Geometry: final body of the model. Coordinates: model frame, mm. Face numbers are marked on the shaded views. Round coordinates to 2 decimals unless told otherwise and drop trailing zeros. Write each loop counter-clockwise with the first axis right and the second up, starting at its lowest first coordinate (ties: lowest second). Pieces come first, ordered by that corner, then holes. Notation, with made-up numbers: (-6.5, 44.25) - (7.5, 44.25) arc R18 cw to (7.5, 68.25) - close; hole circle Ø4 at (61, -4). An arc over 180 degrees is marked (long way). Use a Markdown table: item, result. Add a question column.
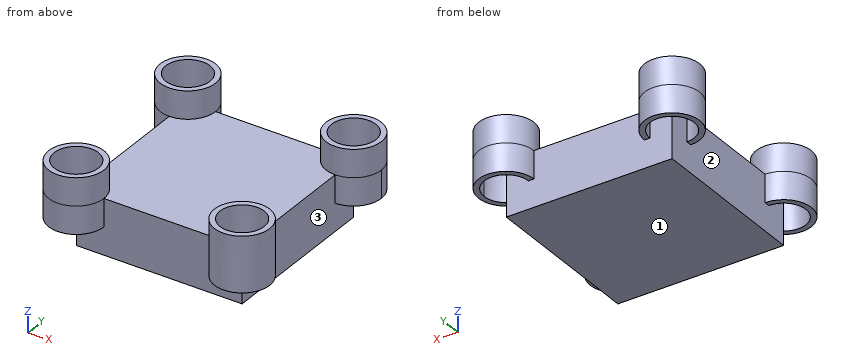
```python
from build123d import *

# Parameters (mm, degrees)
F0_W     = 76.2
F0_H     = 76.2
F1_DEPTH = 25.4
F2_R     = 12.7
F2_R_2   = 10.16
F3_DEPTH = 12.7


with BuildPart() as f1:
    # F0 (on Top) → F1 (new body)
    with BuildSketch(Plane.XY):
        Rectangle(F0_W, F0_H)
    extrude(amount=F1_DEPTH)

    # F2 (on face) → F3 (join, symmetric)
    with BuildSketch(Plane.XY.offset(25.4)):
        with Locations((-38.1, 38.1)):
            Circle(F2_R)
        with Locations((-38.1, 38.1)):
            Circle(F2_R_2, mode=Mode.SUBTRACT)
        with Locations((38.1, 38.1)):
            Circle(F2_R)
        with Locations((38.1, 38.1)):
            Circle(F2_R_2, mode=Mode.SUBTRACT)
        with Locations((-38.1, -38.1)):
            Circle(F2_R)
        with Locations((-38.1, -38.1)):
            Circle(F2_R_2, mode=Mode.SUBTRACT)
        with Locations((38.1, -38.1)):
            Circle(F2_R)
        with Locations((38.1, -38.1)):
            Circle(F2_R_2, mode=Mode.SUBTRACT)
    extrude(amount=F3_DEPTH, both=True)


solid = f1.part
```
1) Draft query along Y for the marked faces 1, 2 and 3. Return one class per face: released by +Y, released by -Y, zero draft, split by the parting line, or undercut.
2) Section C-C, the plane x = 40.5. Return the cut outline in (y, z).
3) Material intervals for L1, parallel to Y at x = -38, z = 21; L2, parallel to X at y = 38, z = 32; L3, parallel to Y at x = -38.5, z = 27, sorted ascending. Write a range as from..to.
4) Section D-D, the plane y = 6.5. Return the cut outline in (x, z), then the cut area to 3 significant figures.
5) Section B-B, the plane y = -33. Return the cut outline in (x, z).
6) Pin query (flat end, axial travel): P1, Ø8, axis at x = 39, y = 14, coming from the +Z side; P2, Ø3, axis at y = -18.5, z = 14.5, coming from the -X side; P3, Ø12.5, axis at x = 11, z = 13.5, coming from the -Y side. Return the tip coordinate at first contact, or that it passes through.
7) Section A-A, the plane z = 31. Return the cut outline in (x, y), then the cut area to 3 significant figures.
Output values:
| question | item | result |
|---|---|---|
| 1 | face 1 | zero draft |
| 1 | face 2 | undercut |
| 1 | face 3 | undercut |
| 2 | outline | (-50.57, 12.7) - (-47.97, 12.7) - (-47.97, 38.1) - (-50.57, 38.1) - close; (-28.23, 12.7) - (-25.63, 12.7) - (-25.63, 38.1) - (-28.23, 38.1) - close; (25.63, 12.7) - (28.23, 12.7) - (28.23, 38.1) - (25.63, 38.1) - close; (47.97, 12.7) - (50.57, 12.7) - (50.57, 38.1) - (47.97, 38.1) - close |
| 3 | L1 | y = -50.8..-48.26, -38.1..38.1, 48.26..50.8 |
| 3 | L2 | x = -50.8..-48.26, -27.94..-25.4, 25.4..27.94, 48.26..50.8 |
| 3 | L3 | y = -50.79..-48.25, -27.95..-25.41, 25.41..27.95, 48.25..50.79 |
| 4 | outline | (-38.1, 0) - (38.1, 0) - (38.1, 25.4) - (-38.1, 25.4) - close |
| 4 | area | 1,940 mm^2 |
| 5 | outline | (-49.73, 12.7) - (-46.89, 12.7) - (-46.89, 38.1) - (-49.73, 38.1) - close; (-38.1, 0) - (38.1, 0) - (38.1, 25.4) - (29.31, 25.4) - (29.31, 38.1) - (26.47, 38.1) - (26.47, 25.4) - (-26.47, 25.4) - (-26.47, 38.1) - (-29.31, 38.1) - (-29.31, 25.4) - (-38.1, 25.4) - close; (46.89, 12.7) - (49.73, 12.7) - (49.73, 38.1) - (46.89, 38.1) - close |
| 6 | P1 | stops at z = 25.4 |
| 6 | P2 | stops at x = -38.1 |
| 6 | P3 | stops at y = -38.1 |
| 7 | outline | circle Ø25.4 at (-38.1, -38.1); circle Ø25.4 at (-38.1, 38.1); circle Ø25.4 at (38.1, -38.1); circle Ø25.4 at (38.1, 38.1); hole circle Ø20.32 at (-38.1, -38.1); hole circle Ø20.32 at (-38.1, 38.1); hole circle Ø20.32 at (38.1, -38.1); hole circle Ø20.32 at (38.1, 38.1) |
| 7 | area | 730 mm^2 |
